Here's the drawing with two shaded views (mm, measured from the low corner). I have some questions. A direction names the side the tool comes from. Round coordinates to 2 decimals unless told otherwise and drop trailing zeros. Loops run counter-clockwise (first coordinate to the right, second up) from the corner with the lowest first, then second, coordinate; pieces in that order, holes last. Notation, with made-up numbers: M -31.75,-22.5 L 21.25,-22.5 A12 ccw 21.25,-2.5 Z; hole C 63,29 d6. An arc over 180 degrees is marked long. One line per item, written item: value. Start each with the question number.
Q1. Imagine slicing it at C-C (x = 25). Please give me the cut outline in (y, z), then the cut area to 3 significant figures.
Q2. Thinking about a two-plate mould opening in X: for the marked faces 1, 2 and 3, which applies, released by +X, released by -X, zero draft, split by the parting line, or undercut?
Q3. Which directions (+Z, -Z, +X, -X, +Y, -Y) give clear straight access to the entire face, cutting with the end or side of a thin tool? Please do the marked faces 4 and 5.
Q4. Imagine slicing it at D-D (y = 28). Please give me the cut outline in (x, z).
Q5. Imagine slicing it at B-B (z = 5). Please give me the cut outline in (x, y), then the cut area to 3 significant figures.
Q6. Please list where these lines run through material, in increasing order: line 1 along Y through (x, z) = (25, 2.5); line 2 along Y through (x, z) = (7, 1.75); line 3 along Y through (x, z) = (36.5, 1.75).
Q7. Imagine slicing it at A-A (y = 35). Please give me the cut outline in (x, z).
Q8. I'm going to push a flat-ended pin straight in: pin 1 Ø2 at (x, z) = (5.5, 5) entering from -Y. Where does the tip first touch, or does it pass through?
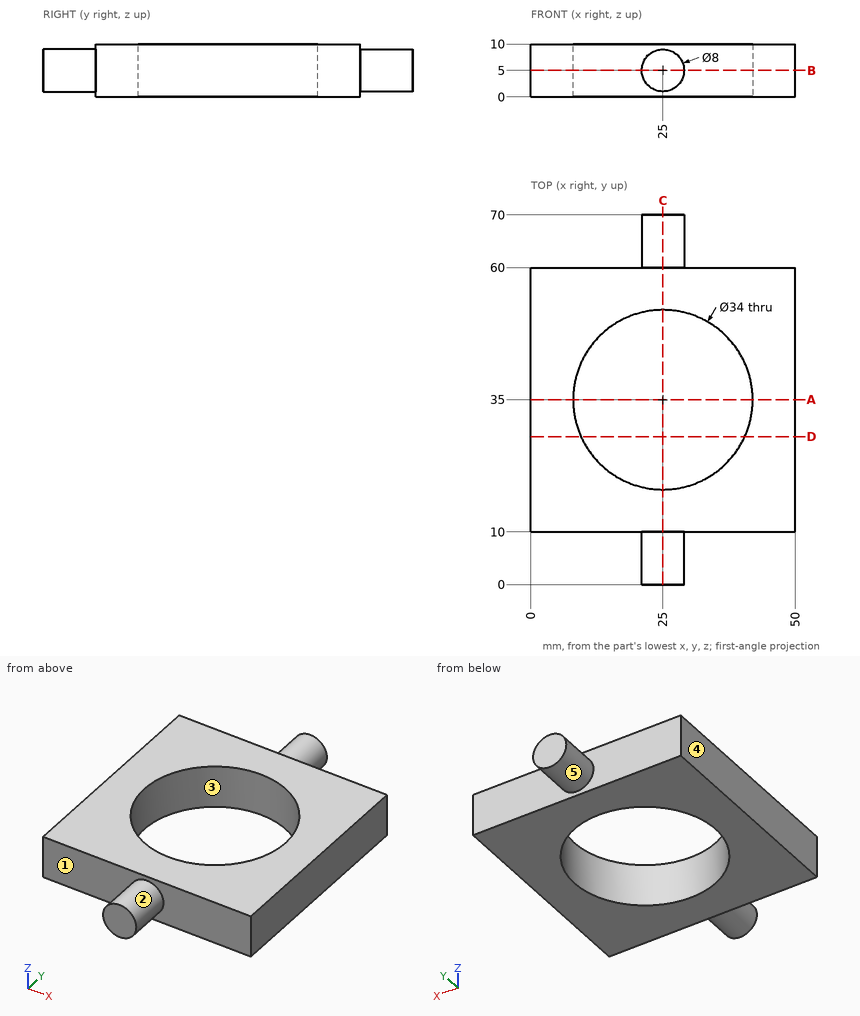
Report:
1. outline: M 0,1 L 10,1 L 10,0 L 18,0 L 18,10 L 10,10 L 10,9 L 0,9 Z; M 52,0 L 60,0 L 60,1 L 70,1 L 70,9 L 60,9 L 60,10 L 52,10 Z
1. area: 320 mm²
2. face 1: zero draft
2. face 2: split by the parting line
2. face 3: undercut
3. face 4: +Z, -Z, -X, +Y, -Y
3. face 5: +Y
4. outline: M 0,0 L 9.51,0 L 9.51,10 L 0,10 Z; M 40.49,0 L 50,0 L 50,10 L 40.49,10 Z
5. outline: M 0,10 L 21,10 L 21,0 L 29,0 L 29,10 L 50,10 L 50,60 L 29,60 L 29,70 L 21,70 L 21,60 L 0,60 Z; hole C 25,35 d34
5. area: 1,750 mm²
6. line 1: y = 0 to 18, 52 to 70
6. line 2: y = 10 to 60
6. line 3: y = 10 to 22.48, 47.52 to 60
7. outline: M 0,0 L 8,0 L 8,10 L 0,10 Z; M 42,0 L 50,0 L 50,10 L 42,10 Z
8. pin 1: stops at y = 10
